Geometry check sheet. Reference: the model listing, model coordinates, mm. A direction names the side the tool comes from. Give positions to 0.01 mm unless a question says otherwise; leave off trailing zeros. Order: outer loops, then holes, each group sorted by start corner. A loop starts at its lowest first (then second) coordinate and runs counter-clockwise, first axis right, second up.
from build123d import *

# Parameters (mm, degrees)
BOSS_EXTRU_1_DEPTH      = 9
ESQUISSE3_R             = 2
BOSS_EXTRU_2_DEPTH      = 1
ESQUISSE4_R             = 2.5
BOSS_EXTRU_3_DEPTH      = 1
BOSS_EXTRU_4_START      = 15
ESQUISSE5_R             = 4
BOSS_EXTRU_4_DEPTH      = 15
BOSS_EXTRU_5_DEPTH      = 9
BOSS_EXTRU_6_DEPTH      = 2
BOSS_EXTRU_6_DEPTH_BACK = 4
ESQUISSE7_R             = 3.8
ESQUISSE8_R             = 5.2
BOSS_EXTRU_7_DEPTH      = 10
ESQUISSE9_R             = 3.2
BOSS_EXTRU_8_DEPTH      = 1
ESQUISSE10_R            = 4.5
BOSS_EXTRU_9_DEPTH      = 1
ESQUISSE11_R            = 2.7
ENL_V_MAT_EXTRU_1_DEPTH = 10
ENL_V_START             = -6
ESQUISSE12_R            = 2.5
ENL_V_MAT_EXTRU_2_DEPTH = 6
CONG_1_R                = 0.4
CHANFREIN1_SIZE         = 1.4


with BuildPart() as part:
    # Esquisse1 → Révolution1 (revolve)
    with BuildSketch(Plane.XY, mode=Mode.PRIVATE) as r_volution1_sk:
        Polygon((-5, 0), (-6, 0), (-4, 1.5), (-4, 3), (-2, 3), (-2, 1.5), align=None)
    revolve(r_volution1_sk.sketch.rotate(Axis((0, 0, 0), (0, 1, 0)), 270), axis=Axis((0, 0, 0), (0, 1, 0)))

    # Esquisse2 → Boss.-Extru.1 (add)
    with BuildSketch(Plane(origin=(0, 3, 0), x_dir=(1, 0, 0), z_dir=(0, 1, 0))):
        Polygon((0, -5.196152423), (4.5, -2.598076211), (4.5, 2.598076211), (0, 5.196152423), (-4.5, 2.598076211), (-4.5, -2.598076211), align=None)
    extrude(amount=BOSS_EXTRU_1_DEPTH)

    # Esquisse3 → Boss.-Extru.2 (add)
    with BuildSketch(Plane(origin=(0, 12, 0), x_dir=(1, 0, 0), z_dir=(0, 1, 0))):
        with Locations(Location((0, 0, 0), (0, 0, 90))):
            Circle(ESQUISSE3_R)
    extrude(amount=BOSS_EXTRU_2_DEPTH)

    # Esquisse4 → Boss.-Extru.3 (add)
    with BuildSketch(Plane(origin=(0, 13, 0), x_dir=(1, 0, 0), z_dir=(0, 1, 0))):
        with Locations(Location((0, 0, 0), (0, 0, 270))):
            Circle(ESQUISSE4_R)
    extrude(amount=BOSS_EXTRU_3_DEPTH)

    # Esquisse5 → Boss.-Extru.4 (add)
    with BuildSketch(Plane(origin=(0, 14, 0), x_dir=(1, 0, 0), z_dir=(0, 1, 0)).offset(BOSS_EXTRU_4_START)):
        with Locations(Location((0, 0, 0), (0, 0, 90))):
            Circle(ESQUISSE5_R)
    extrude(amount=-BOSS_EXTRU_4_DEPTH)

    # Esquisse6 → Boss.-Extru.5 (add)
    with BuildSketch(Plane(origin=(0, 29, 0), x_dir=(1, 0, 0), z_dir=(0, 1, 0))):
        Polygon((4.5, -2.598076211), (4.5, 2.598076211), (0, 5.196152423), (-4.5, 2.598076211), (-4.5, -2.598076211), (0, -5.196152423), align=None)
    extrude(amount=BOSS_EXTRU_5_DEPTH)

    # Esquisse7 → Boss.-Extru.6 (add, two sides: drawn at the far end of the back side and taken through both)
    with BuildSketch(Plane(origin=(4, 0, 0), x_dir=(0, 0, -1), z_dir=(1, 0, 0)).offset(-BOSS_EXTRU_6_DEPTH_BACK)):
        with Locations((0, 21.9)):
            Circle(ESQUISSE7_R)
    extrude(amount=BOSS_EXTRU_6_DEPTH + BOSS_EXTRU_6_DEPTH_BACK)

    # Esquisse8 → Boss.-Extru.7 (add)
    with BuildSketch(Plane(origin=(6, 0, 0), x_dir=(0, 0, -1), z_dir=(1, 0, 0))):
        with Locations((0, 21.9)):
            Circle(ESQUISSE8_R)
    extrude(amount=BOSS_EXTRU_7_DEPTH)

    # Esquisse9 → Boss.-Extru.8 (add)
    with BuildSketch(Plane(origin=(16, 0, 0), x_dir=(0, 0, -1), z_dir=(1, 0, 0))):
        with Locations((0, 21.9)):
            Circle(ESQUISSE9_R)
    extrude(amount=BOSS_EXTRU_8_DEPTH)

    # Esquisse10 → Boss.-Extru.9 (add)
    with BuildSketch(Plane(origin=(17, 0, 0), x_dir=(0, 0, -1), z_dir=(1, 0, 0))):
        with Locations((0, 21.89789892)):
            Circle(ESQUISSE10_R)
    extrude(amount=BOSS_EXTRU_9_DEPTH)

    # Esquisse11 → Enlèv. mat.-Extru.1 (cut)
    with BuildSketch(Plane(origin=(18, 0, 0), x_dir=(0, 0, -1), z_dir=(1, 0, 0))):
        with Locations((0, 21.9)):
            Circle(ESQUISSE11_R)
    extrude(amount=-ENL_V_MAT_EXTRU_1_DEPTH, mode=Mode.SUBTRACT)

    # Esquisse12 → Enlèv. mat.-Extru.2 (cut)
    with BuildSketch(Plane(origin=(0, 38, 0), x_dir=(1, 0, 0), z_dir=(0, 1, 0)).offset(ENL_V_START)):
        with Locations(Location((0, 0, 0), (0, 0, 270))):
            Circle(ESQUISSE12_R)
    extrude(amount=ENL_V_MAT_EXTRU_2_DEPTH, mode=Mode.SUBTRACT)

    # Congé1
    cong_1_edges = [part.edges().sort_by_distance(p)[0] for p in [
        (-2.25, 3, 3.897114317),
        (2.25, 3, 3.897114317),
        (4.5, 3, 0),
        (2.25, 3, -3.897114317),
        (-2.25, 3, -3.897114317),
        (-4.5, 3, 0),
        (-2.25, 12, 3.897114317),
        (2.25, 12, 3.897114317),
        (4.5, 12, 0),
        (2.25, 12, -3.897114317),
        (-2.25, 12, -3.897114317),
        (-4.5, 12, 0),
        (2.25, 29, 3.897114317),
        (4.5, 29, 0),
        (2.25, 29, -3.897114317),
        (-2.25, 29, -3.897114317),
        (-4.5, 29, 0),
        (-2.25, 29, 3.897114317),
        (2.25, 38, 3.897114317),
        (4.5, 38, 0),
        (2.25, 38, -3.897114317),
        (-2.25, 38, -3.897114317),
        (-4.5, 38, 0),
        (-2.25, 38, 3.897114317),
    ]]
    fillet(cong_1_edges, radius=CONG_1_R)

    # Chanfrein1
    chanfrein1_edges = [part.edges().sort_by_distance(p)[0] for p in [
        (6, 21.9, 5.2),
    ]]
    chamfer(chanfrein1_edges, length=CHANFREIN1_SIZE - 0.0001)  # a hair under: the kernel refuses the full size


solid = part.part
Item 1: Draft check along Z on faces 1 (the flat face through (-4.5, 7, 0)), 2 (the cylindrical face through (-2.16, 37.88, 3.82)), 3 (the cylindrical face through (13.07, 24.577, 0.351)), 4 (the cylindrical face through (-2.22, 11.89, -3.77)). Enter one of: released by +Z, released by -Z, zero draft, split by the parting line, or undercut.
Reported:
face 1: zero draft
face 2: released by +Z
face 3: undercut
face 4: released by -Z
Item 2: Sectioned sample at B-B (y = 10). Enter the section's corners in (x, z), and give its area (3 significant figures).
Reported:
outline: (-4.5, -2.6) - (0, -5.2) - (4.5, -2.6) - (4.5, 2.6) - (0, 5.2) - (-4.5, 2.6) - close
area: 70.1 mm2
Item 3: Sectioned sample at A-A (x = 15). Enter the section's corners in (y, z).
Reported:
outline: circle Ø10.4 at (21.9, 0); hole circle Ø5.4 at (21.9, 0)
Item 4: Scan lines: L1, parallel to X at y = 36.2, z = 0; L2, parallel to Y at x = 10.5, z = 0; L3, parallel to X at y = 2.25, z = 0. Record each from-to range of solid material in increasing order.
Reported:
L1: x = -4.5 to -2.5, 2.5 to 4.5
L2: y = 16.7 to 19.2, 24.6 to 27.1
L3: x = -4 to -2, 2 to 4
Item 5: Set-up check for faces 5 (the cylindrical face through (-2.22, 3.12, -3.78)), 6 (the flat face through (0, 32, 0)), 7 (the cylindrical face through (2.22, 11.89, 3.77)), 8 (the cylindrical face through (2.158, 11.886, -3.811)), 9 (the flat face through (0, 3, 4.2)): record each of +Z, -Z, +X, -X, +Y, -Y from which the full face is reachable in a straight line by a thin tool's end or side.
Reported:
face 5: -Z, -X
face 6: +Y
face 7: +Z, +X
face 8: -Z, +X
face 9: none
Item 6: Gauge pin test, flat ends, axial feed: pin 1 (8 mm diameter, centred on x = 14, y = 34, fed in from -Z); pin 2 (5.5 mm diameter, centred on y = 7, z = 1, fed in from -X); pin 3 (4 mm diameter, centred on x = -0.5, z = 1, fed in from -Y); pin 4 (7 mm diameter, centred on y = 20.5, z = -1, fed in from -X). Record the tip position at first contact, or that the pin passes through.
Reported:
pin 1: passes through
pin 2: stops at x = -4.5
pin 3: stops at y = 0.94
pin 4: stops at x = -4
